The listing builds one solid part. Answer for the finished solid, in the listing's coordinates (mm). Face numbers are marked on the shaded views. A direction names the side the tool comes from. Round coordinates to 2 decimals unless told otherwise and drop trailing zeros. Order: outer loops, then holes, each group sorted by start corner. A loop starts at its lowest first (then second) coordinate and runs counter-clockwise, first axis right, second up. Notation, with made-up numbers: (-22.75, 48.5) - (-15.75, 48.5) arc R20 cw to (-15.75, 64.5) - close; hole circle Ø10 at (49, -2). An arc over 180 degrees is marked (long way). One line per item, written item: value. Start each with the question number.
1. Straight lines are drawn through the part: line 1 (Z direction, x = 25, y = 209.55) (3 decimals); line 2 (Z direction, x = -14, y = 450); line 3 (Z direction, x = -34, y = -275). For each, find the intervals that lie inside material, in ascending order.
2. Flat-ended cylindrical pins translate along their axes: P1, Ø11, axis at y = 450.85, z = 31.75, coming from the +X side; P2, Ø5, axis at x = 46.5, z = 108.5, coming from the +Y side; P3, Ø8.5, axis at y = 450.85, z = 95.25, coming from the +X side; P4, Ø5, axis at x = -33, y = -242, coming from the -Z side. Find the tip coordinate at first contact, or state that the pin passes through.
3. Section D-D, the plane x = 12 is taken. Count the separate pieces of the cut face and the enclosed holes in it, then the cut area to 3 significant figures.
4. Section C-C, the plane z = 114 is taken. Give the vertices of the cut face in (x, y).
5. A tool of negligible diameter and unlimited length cuts with its end or side. For the marked faces 1 and 2, from which of +Z, -Z, +X, -X, +Y, -Y can it reach the whole face along a straight path? Write none if from no direction.
6. Section A-A, the plane y = -146.05 is taken. Give the vertices of the cut face in (x, z) (3 decimals).
7. Section B-B, the plane x = -53.5 is taken. Give the vertices of the cut face in (y, z) (3 decimals), then the cut area to 3 significant figures.
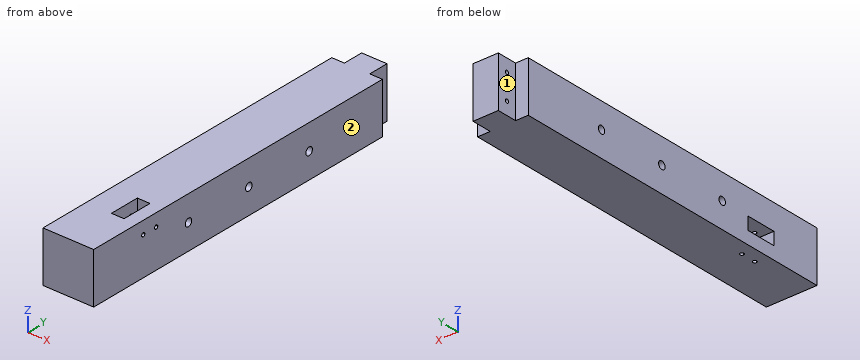
from build123d import *

# Parameters (mm, degrees)
SKETCH1_W           = 63.5
SKETCH1_H           = 50.8
BOSS_EXTRUDE1_DEPTH = 127
SKETCH2_W           = 31.75
SKETCH2_H           = 76.2
CUT_EXTRUDE1_DEPTH  = 63.5
SKETCH3_W           = 31.75
SKETCH3_H           = 76.2
CUT_EXTRUDE3_DEPTH  = 63.246
SKETCH4_R           = 9.525
CUT_EXTRUDE4_DEPTH  = 509.991220455
CUT_EXTRUDE5_DEPTH  = 69.85
CUT_EXTRUDE6_DEPTH  = 69.85
SKETCH7_R           = 4.7625
CUT_EXTRUDE7_DEPTH  = 503.011578552


with BuildPart() as part:
    # Sketch1 → Boss-Extrude1 (new body)
    with BuildSketch(Plane.XY):
        Polygon((63.5, -425.45), (63.5, 425.45), (31.75, 425.45), (31.75, 374.65), (-31.75, 374.65), (-31.75, 425.45), (-63.5, 425.45), (-63.5, -425.45), align=None)
        with Locations((0, 400.05)):
            Rectangle(SKETCH1_W, SKETCH1_H)
        with Locations((0, 450.85)):
            Rectangle(SKETCH1_W, SKETCH1_H)
    extrude(amount=BOSS_EXTRUDE1_DEPTH)

    # Sketch2 → Cut-Extrude1 (cut)
    with BuildSketch(Plane.XY.offset(127)):
        with Locations((15.875, -260.35)):
            Rectangle(SKETCH2_W, SKETCH2_H)
    extrude(amount=-CUT_EXTRUDE1_DEPTH, mode=Mode.SUBTRACT)

    # Sketch3 → Cut-Extrude3 (cut)
    with BuildSketch(Plane.ZY.offset(63.5)):
        with Locations((47.625, -260.35)):
            Rectangle(SKETCH3_W, SKETCH3_H)
    extrude(amount=-CUT_EXTRUDE3_DEPTH, mode=Mode.SUBTRACT)

    # Sketch4 → Cut-Extrude4 (cut, through all)
    with BuildSketch(Plane.ZY.offset(63.5)):
        with Locations(Location((63.5, -146.05, 0), (0, 0, 270))):
            Circle(SKETCH4_R)
        with Locations(Location((63.5, 31.75, 0), (0, 0, 270))):
            Circle(SKETCH4_R)
        with Locations(Location((63.5, 209.55, 0), (0, 0, 270))):
            Circle(SKETCH4_R)
    extrude(amount=-CUT_EXTRUDE4_DEPTH, mode=Mode.SUBTRACT)

    # Sketch5 → Cut-Extrude5 (cut)
    with BuildSketch(Plane(origin=(0, 0, 0), x_dir=(-1, 0, 0), z_dir=(0, 0, -1))):
        with BuildLine():
            ThreePointArc((36.5125, -279.4), (35.117596045, -276.032403955), (31.75, -274.6375))
            Line((31.75, -274.6375), (31.75, -284.1625))
            ThreePointArc((31.75, -284.1625), (35.117596045, -282.767596045), (36.5125, -279.4))
        make_face()
        with BuildLine():
            Line((31.75, -284.1625), (31.75, -274.6375))
            ThreePointArc((31.75, -274.6375), (26.9875, -279.4), (31.75, -284.1625))
        make_face()
        with BuildLine():
            ThreePointArc((36.5125, -241.3), (35.117596045, -237.932403955), (31.75, -236.5375))
            Line((31.75, -236.5375), (31.75, -246.0625))
            ThreePointArc((31.75, -246.0625), (35.117596045, -244.667596045), (36.5125, -241.3))
        make_face()
        with BuildLine():
            Line((31.75, -246.0625), (31.75, -236.5375))
            ThreePointArc((31.75, -236.5375), (26.9875, -241.3), (31.75, -246.0625))
        make_face()
    extrude(amount=-CUT_EXTRUDE5_DEPTH, mode=Mode.SUBTRACT)

    # Sketch6 → Cut-Extrude6 (cut)
    with BuildSketch(Plane(origin=(63.5, 0, 0), x_dir=(0, 0, -1), z_dir=(1, 0, 0))):
        with BuildLine():
            ThreePointArc((-90.4875, -241.3), (-91.882403955, -237.932403955), (-95.25, -236.5375))
            Line((-95.25, -236.5375), (-95.25, -246.0625))
            ThreePointArc((-95.25, -246.0625), (-91.882403955, -244.667596045), (-90.4875, -241.3))
        make_face()
        with BuildLine():
            Line((-95.25, -246.0625), (-95.25, -236.5375))
            ThreePointArc((-95.25, -236.5375), (-100.0125, -241.3), (-95.25, -246.0625))
        make_face()
        with BuildLine():
            ThreePointArc((-90.4875, -279.4), (-91.882403955, -276.032403955), (-95.25, -274.6375))
            Line((-95.25, -274.6375), (-95.25, -284.1625))
            ThreePointArc((-95.25, -284.1625), (-91.882403955, -282.767596045), (-90.4875, -279.4))
        make_face()
        with BuildLine():
            Line((-95.25, -284.1625), (-95.25, -274.6375))
            ThreePointArc((-95.25, -274.6375), (-100.0125, -279.4), (-95.25, -284.1625))
        make_face()
    extrude(amount=-CUT_EXTRUDE6_DEPTH, mode=Mode.SUBTRACT)

    # Sketch7 → Cut-Extrude7 (cut, through all)
    with BuildSketch(Plane(origin=(31.75, 0, 0), x_dir=(0, 0, -1), z_dir=(1, 0, 0))):
        with Locations(Location((-95.25, 450.85, 0), (0, 0, 90))):
            Circle(SKETCH7_R)
        with Locations(Location((-31.75, 450.85, 0), (0, 0, 90))):
            Circle(SKETCH7_R)
    extrude(amount=-CUT_EXTRUDE7_DEPTH, mode=Mode.SUBTRACT)


solid = part.part
Answer list:
1. line 1: z = 0 to 53.975, 73.025 to 127
1. line 2: z = 0 to 27.06, 36.44 to 90.56, 99.94 to 127
1. line 3: z = 0 to 31.75, 63.5 to 127
2. P1: stops at x = 31.75
2. P2: stops at y = 425.45
2. P3: passes through
2. P4: stops at z = 69.85
3. separate pieces: 1
3. enclosed holes: 5
3. area: 109,000 mm²
4. outline: (-63.5, -425.45) - (63.5, -425.45) - (63.5, 425.45) - (31.75, 425.45) - (31.75, 476.25) - (-31.75, 476.25) - (-31.75, 425.45) - (-63.5, 425.45) - close; hole (0, -298.45) - (31.75, -298.45) - (31.75, -222.25) - (0, -222.25) - close
5. face 1: +Z, -Z, -X, +Y
5. face 2: +Z, -Z, +X, +Y, -Y
6. outline: (-63.5, 0) - (63.5, 0) - (63.5, 53.975) - (-63.5, 53.975) - close; (-63.5, 73.025) - (63.5, 73.025) - (63.5, 127) - (-63.5, 127) - close
7. outline: (-425.45, 0) - (425.45, 0) - (425.45, 127) - (-425.45, 127) - close; hole (-298.45, 31.75) - (-222.25, 31.75) - (-222.25, 63.5) - (-298.45, 63.5) - close; hole circle Ø19.05 at (-146.05, 63.5); hole circle Ø19.05 at (31.75, 63.5); hole circle Ø19.05 at (209.55, 63.5)
7. area: 105,000 mm²
